Can you work these out from the model? Positions are in its coordinate system, mm. Face numbers are marked on the shaded views. Coordinates: 2 decimals unless noted, no trailing zeros. Loops run counter-clockwise (first coordinate to the right, second up) from the corner with the lowest first, then second, coordinate; pieces in that order, holes last. Notation, with made-up numbers: M 51,20 L 85,20 A26 ccw 85,46 Z; hole C 55,-5.75 d2. An arc over 180 degrees is marked long. Answer as a JSON object with one key per item and string values. Group by question number.
Item 1: We'd pull the mould along X, two halves only. Please class the marked faces 1 and 2: +X half, -X half, draft (parallel to the pull), parting line (faces both ways), or undercut.
Item 2: Suppose I cut it at C-C (z = 346). Write out the boundary of the cut face in (x, y), then the cut area to 3 significant figures.
Item 3: I'm going to push flat-ended pins straight in: pin 1 Ø0.8 at (x, y) = (0.5, -17) entering from -Z; pin 2 Ø3 at (x, y) = (-14, 11) entering from +Z; pin 3 Ø1.3 at (y, z) = (-17, 197) entering from +X; pin 4 Ø1.8 at (y, z) = (-16.5, 195) entering from -X. Where does each tip first touch, or does it pass through?
Item 4: If I drill on line 1 (X direction, y = -10.5, z = 202); line 2 (X direction, y = -10, z = 12.5), over which ranges is the centre line in solid material (lowest first)?
Item 5: Suppose I cut it at D-D (z = 190.5). Write out the boundary of the cut face in (x, y), then the cut area to 3 significant figures.
Item 6: Suppose I cut it at A-A (y = -2). Write out the boundary of the cut face in (x, z).
Item 7: Suppose I cut it at B-B (x = 3). Write out the boundary of the cut face in (y, z), then the cut area to 3 significant figures.
Autodesk Inventor part; units mm, degrees
ref_plane "Start plane" through (0, 0, -17.5) normal (0, 0, 1) x (1, 0, 0)
ref_plane "End plane" through (0, 0, 405.5) normal (0, 0, 1) x (1, 0, 0)
ref_plane "Work Plane4" through (0, 0, 194) normal (0, -1, 0) x (1, 0, 0)
ref_plane "Start plane" through (0, 0, -17.5) normal (0, 0, 1) x (1, 0, 0)
ref_plane "End plane" through (0, 0, 405.5) normal (0, 0, 1) x (1, 0, 0)
sketch "Sketch" plane through (0, 0, 0) normal (0, 0, 1) x (1, 0, 0)
  line L0 (-17.5, -14.3) -> (-17.5, 14.3)
  line L1 (-14.3, 17.5) -> (14.3, 17.5)
  line L2 (17.5, 14.3) -> (17.5, -14.3)
  line L3 (14.3, -17.5) -> (-14.3, -17.5)
  arc A0 (-17.5, -14.3) -> (-14.3, -17.5) centre (-14.3, -14.3) ccw
  arc A1 (-14.3, 17.5) -> (-17.5, 14.3) centre (-14.3, 14.3) ccw
  arc A2 (17.5, 14.3) -> (14.3, 17.5) centre (14.3, 14.3) ccw
  arc A3 (14.3, -17.5) -> (17.5, -14.3) centre (14.3, -14.3) ccw
  arc A4 (-14.3, 15.9) -> (-15.9, 14.3) centre (-14.3, 14.3) ccw
  line L4 (-14.3, 15.9) -> (14.3, 15.9)
  arc A5 (15.9, 14.3) -> (14.3, 15.9) centre (14.3, 14.3) ccw
  line L5 (15.9, 14.3) -> (15.9, -14.3)
  arc A6 (14.3, -15.9) -> (15.9, -14.3) centre (14.3, -14.3) ccw
  line L6 (14.3, -15.9) -> (-14.3, -15.9)
  arc A7 (-15.9, -14.3) -> (-14.3, -15.9) centre (-14.3, -14.3) ccw
  line L7 (-15.9, -14.3) -> (-15.9, 14.3)
  line L8 (0, 25.4278) -> (0, -25.4278) construction
  line L9 (-25.4278, 0) -> (25.4278, 0) construction
  dimension "d7" = 3.2
  dimension "d10" = 35
  dimension "d11" = 35
  dimension "d12" = 1.6
  dimension "d15" = 17.5
  dimension "d16" = 17.5
extrude "Body" add sketch "Sketch" along normal up to surface (423 mm away) from surface at -17.5
sketch "Sketch3" plane through (0, 0, 0) normal (0, 0, 1) x (1, 0, 0)
  line L0 (0, 0) -> (10, 0)
ref_plane "Work Plane3" through (0, 0, 0) normal (0, -1, 0) x (1, 0, 0)
sketch "Sketch4" plane through (0, 0, 0) normal (0, -1, 0) x (1, 0, 0)
  line L0 (-2, -17.5) -> (12, -17.5)
  line L1 (-2, 405.5) -> (12, 405.5)
  dimension "d18" = 423
ref_plane "Work Plane4" through (0, 0, 194) normal (0, -1, 0) x (1, 0, 0)
ref_plane "Work Plane5" through (0, -150, 194) normal (0, -1, 0) x (1, 0, 0)
ref_plane "Work Plane6" through (0, -75, 194) normal (0, -1, 0) x (1, 0, 0)
sketch "Sketch5" plane through (0, -75, 194) normal (0, -1, 0) x (1, 0, 0)
  arc A0 (-12.5, -9.3) -> (-9.3, -12.5) centre (-9.3, -9.3) ccw
  line L0 (-12.5, -9.3) -> (-12.5, 9.3)
  arc A1 (-9.3, 12.5) -> (-12.5, 9.3) centre (-9.3, 9.3) ccw
  line L1 (-9.3, 12.5) -> (9.3, 12.5)
  arc A2 (12.5, 9.3) -> (9.3, 12.5) centre (9.3, 9.3) ccw
  line L2 (12.5, 9.3) -> (12.5, -9.3)
  arc A3 (9.3, -12.5) -> (12.5, -9.3) centre (9.3, -9.3) ccw
  line L3 (9.3, -12.5) -> (-9.3, -12.5)
  arc A4 (-9.3, 10.9) -> (-10.9, 9.3) centre (-9.3, 9.3) ccw
  line L4 (-9.3, 10.9) -> (9.3, 10.9)
  arc A5 (10.9, 9.3) -> (9.3, 10.9) centre (9.3, 9.3) ccw
  line L5 (10.9, 9.3) -> (10.9, -9.3)
  arc A6 (9.3, -10.9) -> (10.9, -9.3) centre (9.3, -9.3) ccw
  line L6 (9.3, -10.9) -> (-9.3, -10.9)
  arc A7 (-10.9, -9.3) -> (-9.3, -10.9) centre (-9.3, -9.3) ccw
  line L7 (-10.9, -9.3) -> (-10.9, 9.3)
extrude "Extrusion2" cut sketch "Sketch5" along normal up to surface (150 mm away) from surface at -75 contours L0 A1 L1 A2 L2 A3 L3 A0 | L4 A5 L5 A6 L6 A7 L7 A4
ref_plane "Work Plane7" through (-12.5983, 0, 400.9862) normal (-0.4912, 0, 0.871) x (0.871, 0, 0.4912)
split "Split1" plane through (-12.5983, 0, 400.9862) removes the side toward (-0.4912, 0, 0.871)
ref_plane "Work Plane8" through (-687.6928, 0, 367.7357) normal (-0.4912, 0, -0.871) x (-0.871, 0, 0.4912)
split "Split2" plane through (-687.6928, 0, 367.7357) removes the side toward (-0.4912, 0, -0.871)
ref_plane "Work Plane9" through (17.5, 0, -17.5) normal (-0.7071, 0, -0.7071) x (-0.7071, 0, 0.7071)
split "Split3" plane through (17.5, 0, -17.5) removes the side toward (-0.7071, 0, -0.7071)
ref_plane "Work Plane10" through (17.5, 0, 405.5) normal (-0.7071, 0, 0.7071) x (0.7071, 0, 0.7071)
split "Split4" plane through (17.5, 0, 405.5) removes the side toward (-0.7071, 0, 0.7071)
equation "\"d7\" = G_IR"
equation "\"d10\" = G_H"
equation "\"d11\" = G_W"
equation "\"d12\" = G_T"
equation "\"d15\" = 0.5 * d10"
equation "\"d16\" = 0.5 * d11"
equation "\"d3\" = G_L"
equation "\"G_W\" = 35"
equation "\"G_H\" = 35"
equation "\"G_T\" = 1.6"
equation "\"G_IR\" = 3.2"
equation "\"G_L\" = d18"
equation "\"G_OFFSET_START\" = 17.5"
equation "\"G_OFFSET_END\" = 17.5"
equation "\"d13\" = -G_OFFSET_START"
equation "\"d14\" = G_OFFSET_END + B_L"
equation "\"B_L\" = 388"
properties part number "AS 1163 - C350L0 35x35x1.6 SHS - 423" material "Steel, Mild"
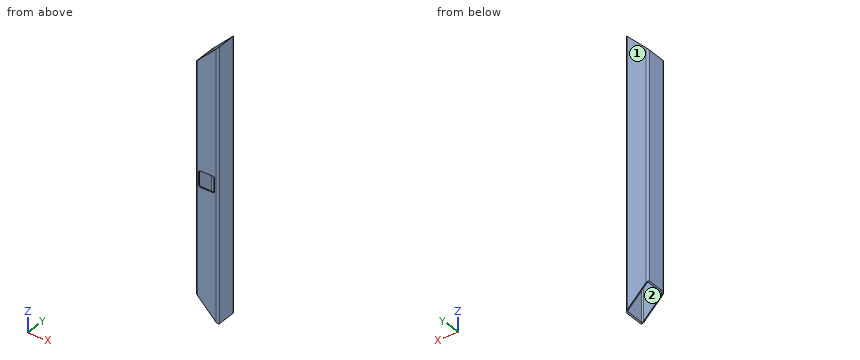
From the geometry:
{
 "1": {"face 1": "draft", "face 2": "undercut"},
 "2": {"outline": "M -17.5,-14.3 A3.2 ccw -14.3,-17.5 L 14.3,-17.5 A3.2 ccw 17.5,-14.3 L 17.5,14.3 A3.2 ccw 14.3,17.5 L -14.3,17.5 A3.2 ccw -17.5,14.3 Z; hole M -15.9,-14.3 A1.6 ccw -14.3,-15.9 L 14.3,-15.9 A1.6 ccw 15.9,-14.3 L 15.9,14.3 A1.6 ccw 14.3,15.9 L -14.3,15.9 A1.6 ccw -15.9,14.3 Z", "area": "207 mm2"},
 "3": {"pin 1": "z = -0.9", "pin 2": "through", "pin 3": "x = 16.76", "pin 4": "x = -17.22"},
 "4": {"line 1": "-17.5 to -15.9, 15.9 to 17.5", "line 2": "15.9 to 17.5"},
 "5": {"outline": "M -17.5,-14.3 A3.2 ccw -14.3,-17.5 L -12.5,-17.5 L -12.5,-15.9 L -14.3,-15.9 A1.6 cw -15.9,-14.3 L -15.9,14.3 A1.6 cw -14.3,15.9 L 14.3,15.9 A1.6 cw 15.9,14.3 L 15.9,-14.3 A1.6 cw 14.3,-15.9 L 12.5,-15.9 L 12.5,-17.5 L 14.3,-17.5 A3.2 ccw 17.5,-14.3 L 17.5,14.3 A3.2 ccw 14.3,17.5 L -14.3,17.5 A3.2 ccw -17.5,14.3 Z", "area": "167 mm2"},
 "6": {"outline": "M -17.5,17.5 L -15.9,15.9 L -15.9,372.1 L -17.5,370.5 Z; M 15.9,-15.9 L 17.5,-17.5 L 17.5,405.5 L 15.9,403.9 Z"},
 "7": {"outline": "M -17.5,-3 L -15.9,-3 L -15.9,181.5 L -17.5,181.5 Z; M -17.5,206.5 L -15.9,206.5 L -15.9,391 L -17.5,391 Z; M 15.9,-3 L 17.5,-3 L 17.5,391 L 15.9,391 Z", "area": "1,220 mm2"}
}
